Part print with two shaded views. Sizes in mm from the minimum x, y, z corner. Coordinates: 2 decimals unless noted, no trailing zeros. Write each loop counter-clockwise with the first axis right and the second up, starting at its lowest first coordinate (ties: lowest second). Pieces come first, ordered by that corner, then holes. Notation, with made-up numbers: (-16, 33.25) - (27, 33.25) arc R16 ccw to (27, 54.25) - close; hole circle Ø10 at (19.25, 26.25). An arc over 180 degrees is marked (long way). One line per question, with ' | ' between items. Start each with the question number.
1. Band-saw the part on B-B, the plane x = 241.3. Give the number of separate pieces and of enclosed holes in the cut face, then the cut area to 3 significant figures.
2. Flat gauge pin, fed straight in: P1, Ø6, axis at x = 292.1, y = 12.7, coming from the +Z side. Where does the tip first touch, or does it go through?
3. Two-plate mould, pull along Z, no slides. Class the marked faces 1, 2, 3 and 4: +Z half, -Z half, draft (parallel to the pull), parting line (faces both ways), or undercut.
4. Band-saw the part on C-C, the plane x = 96. Write the cut outline in (y, z) (1 decimal).
5. Probe line 1 (Y direction, x = 267, z = 1.75) (1 decimal); line 2 (Y direction, x = 139.7, z = 1.9); line 3 (Z direction, x = 215, y = 42.5) (1 decimal). List the from-to ranges inside material, lowest first.
6. Band-saw the part on A-A, the plane y = 30. Write the cut outline in (x, z) (1 decimal).
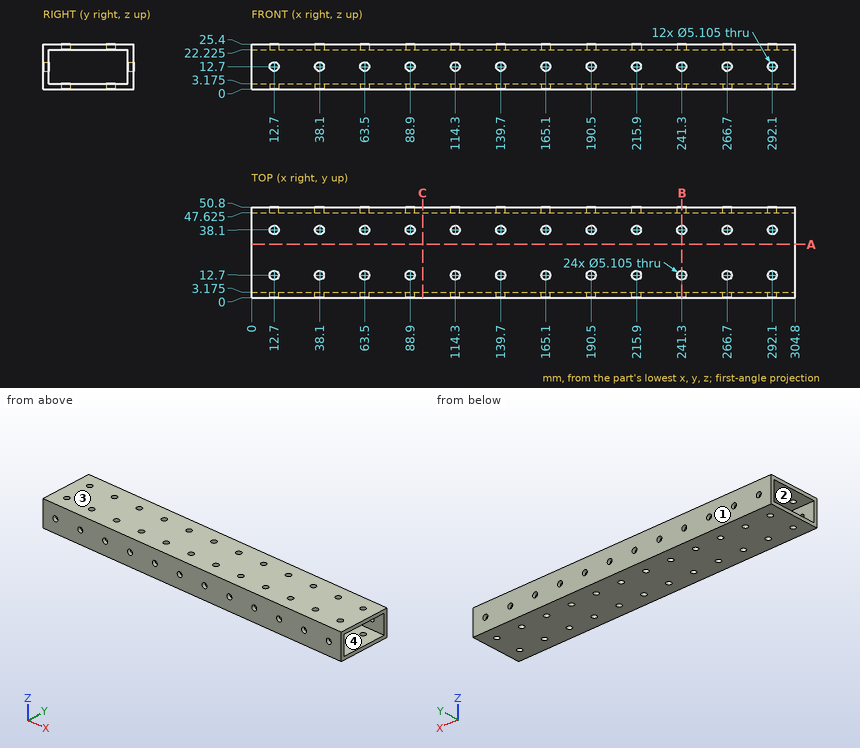
Filled in:
1) separate pieces: 6 | enclosed holes: 0 | area: 346 mm²
2) P1: stops at z = 25.4
3) face 1: draft | face 2: undercut | face 3: +Z half | face 4: undercut
4) outline: (0, 0) - (50.8, 0) - (50.8, 25.4) - (0, 25.4) - close; hole (3.2, 3.2) - (47.6, 3.2) - (47.6, 22.2) - (3.2, 22.2) - close
5) line 1: y = 0 to 10.2, 15.2 to 35.6, 40.6 to 50.8 | line 2: y = 0 to 10.15, 15.25 to 35.55, 40.65 to 50.8 | line 3: z = 0 to 3.2, 22.2 to 25.4
6) outline: (0, 0) - (304.8, 0) - (304.8, 3.2) - (0, 3.2) - close; (0, 22.2) - (304.8, 22.2) - (304.8, 25.4) - (0, 25.4) - close
